```python
from build123d import *

# Parameters (mm, degrees)
BOSS_EXTRUDE1_DEPTH     = 3.175
SKETCH2_W               = 3.175
SKETCH2_H               = 3.175
CUT_EXTRUDE1_DEPTH      = 1
CUT_EXTRUDE1_DEPTH_BACK = 4.175


with BuildPart() as part:
    # Sketch1 → Boss-Extrude1 (new body)
    with BuildSketch(Plane.XY):
        with BuildLine():
            Line((15.24, 15.7607), (50.165, 15.7607))
            ThreePointArc((50.165, 15.7607), (52.41006403, 16.69063597), (53.34, 18.9357))
            Line((53.34, 18.9357), (53.34, 26.8732))
            ThreePointArc((53.34, 26.8732), (52.41006403, 29.11826403), (50.165, 30.0482))
            Line((50.165, 30.0482), (3.175, 30.0482))
            ThreePointArc((3.175, 30.0482), (0.92993597, 29.11826403), (0, 26.8732))
            Line((0, 26.8732), (0, 17.78))
            Line((0, 17.78), (-44.45, 17.78))
            Line((-44.45, 17.78), (-44.45, 26.8732))
            ThreePointArc((-44.45, 26.8732), (-45.37993597, 29.11826403), (-47.625, 30.0482))
            Line((-47.625, 30.0482), (-53.975, 30.0482))
            ThreePointArc((-53.975, 30.0482), (-56.22006403, 29.11826403), (-57.15, 26.8732))
            Line((-57.15, 26.8732), (-57.15, -4.8768))
            ThreePointArc((-57.15, -4.8768), (-56.22006403, -7.12186403), (-53.975, -8.0518))
            Line((-53.975, -8.0518), (-47.625, -8.0518))
            ThreePointArc((-47.625, -8.0518), (-45.37993597, -7.12186403), (-44.45, -4.8768))
            Line((-44.45, -4.8768), (-44.45, 0))
            Line((-44.45, 0), (0, 0))
            Line((0, 0), (0, -4.8768))
            ThreePointArc((0, -4.8768), (0.92993597, -7.12186403), (3.175, -8.0518))
            Line((3.175, -8.0518), (50.165, -8.0518))
            ThreePointArc((50.165, -8.0518), (52.41006403, -7.12186403), (53.34, -4.8768))
            Line((53.34, -4.8768), (53.34, 3.0607))
            ThreePointArc((53.34, 3.0607), (52.41006403, 5.30576403), (50.165, 6.2357))
            Line((50.165, 6.2357), (15.24, 6.2357))
            ThreePointArc((15.24, 6.2357), (10.4775, 10.9982), (15.24, 15.7607))
        make_face()
    extrude(amount=BOSS_EXTRUDE1_DEPTH)

    # Sketch2 → Cut-Extrude1 (cut, two sides)
    with BuildSketch(Plane.XY.offset(3.175)) as cut_extrude1_sk:
        with Locations((26.67, -4.8768)):
            Rectangle(SKETCH2_W, SKETCH2_H)
        with Locations((-50.8, 26.8732)):
            Rectangle(SKETCH2_W, SKETCH2_H)
        with Locations((26.67, 26.8732)):
            Rectangle(SKETCH2_W, SKETCH2_H)
        with Locations((-50.8, -4.8768)):
            Rectangle(SKETCH2_W, SKETCH2_H)
    extrude(amount=CUT_EXTRUDE1_DEPTH, mode=Mode.SUBTRACT)
    extrude(cut_extrude1_sk.sketch, amount=-CUT_EXTRUDE1_DEPTH_BACK, mode=Mode.SUBTRACT)


solid = part.part
```
Work out the finished part from the listing and answer in its coordinate system (mm). A direction names the side the tool comes from. Coordinates: 2 decimals unless noted, no trailing zeros. Order: outer loops, then holes, each group sorted by start corner. A loop starts at its lowest first (then second) coordinate and runs counter-clockwise, first axis right, second up. Notation, with made-up numbers: M 59,-18 L 110,-18 A22 ccw 110,0 Z; hole C -15.5,26 d4. An arc over 180 degrees is marked long. Use CSV: the item, a comma, the result in double quotes.
1) Determine the mould class of faces 6 (the face through (52.435, 5.281, 1.565)), 7 (the face through (27, -6.464, 2)), 8 (the face through (-51, -8.052, 2)) for opening direction X: released by +X, released by -X, zero draft, split by the parting line, or undercut.
Worked out:
face 6,"released by +X"
face 7,"undercut"
face 8,"zero draft"
2) Section C-C on y = 9 is taken. Write down the section's boundary in (x, z) (3 decimals), plus the area to 3 significant figures.
Worked out:
outline,"M -57.15,0 L 10.917,0 L 10.917,3.175 L -57.15,3.175 Z"
area,"216 mm^2"
3) For faces 1 (the face through (-45.405, -7.146, 1.565)), 2 (the face through (-44.45, 22, 2)), 3 (the face through (-49.212, -5, 2)), 4 (the face through (53.34, 23, 2)), 5 (the face through (52.435, 29.093, 1.565)), determine the directions among +Z, -Z, +X, -X, +Y, -Y from which every point of the face is accessible in a straight line to the end or side of a thin tool.
Worked out:
face 1,"+Z, -Z, -Y"
face 2,"+Z, -Z, +Y"
face 3,"+Z, -Z"
face 4,"+Z, -Z, +X, +Y, -Y"
face 5,"+Z, -Z, +X, +Y"
4) Section A-A on x = 42.5 is taken. Write down the section's boundary in (y, z) (3 decimals).
Worked out:
outline,"M -8.052,0 L 6.236,0 L 6.236,3.175 L -8.052,3.175 Z; M 15.761,0 L 30.048,0 L 30.048,3.175 L 15.761,3.175 Z"
5) Consider line 1 (Y direction, x = 36.5, z = 2.35); line 2 (X direction, y = -4, z = 0.9); line 3 (Y direction, x = -16, z = 0.8). Determine where each line is inside the solid, lowest interval first. Write a range as [from, to].
Worked out:
line 1,"y = [-8.05, 6.24], [15.76, 30.05]"
line 2,"x = [-57.15, -52.39], [-49.21, -44.45], [0, 25.08], [28.26, 53.34]"
line 3,"y = [0, 17.78]"
6) Section B-B on z = 1.95 is taken. Count the separate pieces of the cut face and the enclosed holes in it, plus the area to 3 significant figures.
Worked out:
separate pieces,"1"
enclosed holes,"4"
area,"2,850 mm^2"
7) Section D-D on y = 14 is taken. Write down the section's boundary in (x, z) (3 decimals), plus the area to 3 significant figures.
Worked out:
outline,"M -57.15,0 L 11.543,0 L 11.543,3.175 L -57.15,3.175 Z"
area,"218 mm^2"
8) A flat-ended cylindrical pin translates along its axis: pin 1 Ø1 at (x, z) = (-9.5, 2.5) entering from +Y. Find the tip coordinate at first contact, or state that the pin passes through.
Worked out:
pin 1,"stops at y = 17.78"
